Autodesk Inventor part; units mm, degrees
ref_plane "YZ Plane" through (0, 0, 0) normal (1, 0, 0) x (0, 1, 0)
ref_plane "XZ Plane" through (0, 0, 0) normal (0, 1, 0) x (-1, 0, 0)
ref_plane "XY Plane" through (0, 0, 0) normal (0, 0, 1) x (1, 0, 0)
sketch "Sketch1" plane through (0, 0, 0) normal (0, 0, 1) x (1, 0, 0)
  circle A0 centre (-11.375, 11.375) radius 2.1
  circle A1 centre (-11.375, -11.375) radius 2.1
  line L0 (-15, 4.1) -> (-12.9, 4.1)
  line L1 (-12.9, 4.1) -> (-12.9, 8.28)
  line L2 (-12.9, 8.28) -> (-9.85, 8.28)
  line L3 (-9.85, 8.28) -> (-5.8, 4.23)
  line L4 (-5.8, 4.23) -> (-5.8, -4.23)
  line L5 (-5.8, -4.23) -> (-9.85, -8.28)
  line L6 (-9.85, -8.28) -> (-12.9, -8.28)
  line L7 (-12.9, -8.28) -> (-12.9, -4.1)
  line L8 (-12.9, -4.1) -> (-15, -4.1)
  line L9 (-15, -4.1) -> (-15, -13)
  arc A2 (-15, -13) -> (-13, -15) centre (-13, -13) ccw
  line L10 (-13, -15) -> (-4.1, -15)
  line L11 (-4.1, -15) -> (-4.1, -12.9)
  line L12 (-4.1, -12.9) -> (-8.28, -12.9)
  line L13 (-8.28, -12.9) -> (-8.28, -9.85)
  line L14 (-8.28, -9.85) -> (-3.719, -5.289)
  line L15 (-3.719, -5.289) -> (3.719, -5.289)
  line L16 (3.719, -5.289) -> (8.28, -9.85)
  line L17 (8.28, -9.85) -> (8.28, -12.9)
  line L18 (8.28, -12.9) -> (4.1, -12.9)
  line L19 (4.1, -12.9) -> (4.1, -15)
  line L20 (4.1, -15) -> (13, -15)
  arc A3 (13, -15) -> (15, -13) centre (13, -13) ccw
  line L21 (15, -13) -> (15, -4.1)
  line L22 (15, -4.1) -> (12.9, -4.1)
  line L23 (12.9, -4.1) -> (12.9, -8.28)
  line L24 (12.9, -8.28) -> (9.85, -8.28)
  line L25 (9.85, -8.28) -> (5.8, -4.23)
  line L26 (5.8, -4.23) -> (5.8, 4.23)
  line L27 (5.8, 4.23) -> (9.85, 8.28)
  line L28 (9.85, 8.28) -> (12.9, 8.28)
  line L29 (12.9, 8.28) -> (12.9, 4.1)
  line L30 (12.9, 4.1) -> (15, 4.1)
  line L31 (15, 4.1) -> (15, 13)
  arc A4 (15, 13) -> (13, 15) centre (13, 13) ccw
  line L32 (13, 15) -> (4.1, 15)
  line L33 (4.1, 15) -> (4.1, 12.9)
  line L34 (4.1, 12.9) -> (8.28, 12.9)
  line L35 (8.28, 12.9) -> (8.28, 9.85)
  line L36 (8.28, 9.85) -> (3.719, 5.289)
  line L37 (3.719, 5.289) -> (-3.719, 5.289)
  line L38 (-3.719, 5.289) -> (-8.28, 9.85)
  line L39 (-8.28, 9.85) -> (-8.28, 12.9)
  line L40 (-8.28, 12.9) -> (-4.1, 12.9)
  line L41 (-4.1, 12.9) -> (-4.1, 15)
  line L42 (-4.1, 15) -> (-13, 15)
  arc A5 (-13, 15) -> (-15, 13) centre (-13, 13) ccw
  line L43 (-15, 13) -> (-15, 4.1)
  circle A6 centre (0, 0) radius 3.4
  circle A7 centre (11.375, 11.375) radius 2.1
  circle A8 centre (11.375, -11.375) radius 2.1
extrude "Extrusion1" add sketch "Sketch1" against normal blind 300
sketch "Sketch2" plane through (-13, 15, 0) normal (0, 1, 0) x (1, 0, 0)
  point P0 (13, 0)
properties part number "Metal Profile 30 cm" material "Aluminum 6061-AHC"
The model under review builds one solid part; all positions refer to its coordinate system, in mm. A direction names the side the tool comes from. Coordinates: 2 decimals unless noted, no trailing zeros. Write each loop counter-clockwise with the first axis right and the second up, starting at its lowest first coordinate (ties: lowest second). Pieces come first, ordered by that corner, then holes. Notation, with made-up numbers: (-13.75, 68.5) - (23.25, 68.5) arc R9 ccw to (23.25, 78.5) - close; hole circle Ø9 at (64.5, -18.5). An arc over 180 degrees is marked (long way). Answer in a Markdown table with one row per item. Add a question column.
Q1. Consider section A-A on x = 0. Give the boundary of the cut face in (y, z), then the cut area to 3 significant figures.
Q2. For faces 1 (the face through (0, -5.289, -148)), 2 (the face through (5.97, -7.54, -147.9)), 3 (the face through (9, 15, -148)), list the 3-axis set-ups (+Z, -Z, +X, -X, +Y, -Y) from which the entire face can be reached by the end or side of a thin tool; tool diameter is ignored.
Q3. Consider section C-C on z = -54.5. Give the number of separate pieces and of enclosed holes in the cut face, then the cut area to 3 significant figures.
Q4. To check wall thickness, follow line 1 along X through (y, z) = (11.5, -195.5); line 2 along X through (y, z) = (-0.25, -203); line 3 along Y through (x, z) = (0, -135). State the ranges of each line that lie inside material, in increasing order. Write a range as from..to.
Q5. Consider section B-B on y = 0. Give the boundary of the cut face in (x, z), then the cut area to 3 significant figures.
Q6. Clearance check with flat-ended pins moving along their axes: pin 1 (3.5 mm diameter, centred on x = 11.375, y = -11.375, fed in from -Z); pin 2 (2.5 mm diameter, centred on y = -14.5, z = -127, fed in from +X); pin 3 (1.7 mm diameter, centred on y = 14, z = -203, fed in from -X); pin 4 (4 mm diameter, centred on y = -0.5, z = -117.5, fed in from -X). State where each tip first meets the part, or that it passes through.
Q7. Draft analysis for pull direction X (two halves, no side actions). For faces 4 (the face through (-4, 0, 0)), 5 (the face through (15, 8, -148)), 6 (the face through (-15, 9, -148)), 7 (the face through (0, 5.289, -148)), state which applies: +X half, -X half, draft (parallel to the pull), parting line (faces both ways), or undercut.
Answers below:
| question | item | result |
|---|---|---|
| 1 | outline | (-5.29, -300) - (-3.4, -300) - (-3.4, 0) - (-5.29, 0) - close; (3.4, -300) - (5.29, -300) - (5.29, 0) - (3.4, 0) - close |
| 1 | area | 1,130 mm² |
| 2 | face 1 | +Z, -Z, -Y |
| 2 | face 2 | +Z, -Z |
| 2 | face 3 | +Z, -Z, +X, -X, +Y |
| 3 | separate pieces | 1 |
| 3 | enclosed holes | 5 |
| 3 | area | 323 mm² |
| 4 | line 1 | -15..-13.47, -9.28..-8.28, 8.28..9.28, 13.47..15 |
| 4 | line 2 | -5.8..-3.39, 3.39..5.8 |
| 4 | line 3 | -5.29..-3.4, 3.4..5.29 |
| 5 | outline | (-5.8, -300) - (-3.4, -300) - (-3.4, 0) - (-5.8, 0) - close; (3.4, -300) - (5.8, -300) - (5.8, 0) - (3.4, 0) - close |
| 5 | area | 1,440 mm² |
| 6 | pin 1 | through |
| 6 | pin 2 | x = 14.98 |
| 6 | pin 3 | x = -14.99 |
| 6 | pin 4 | x = -5.8 |
| 7 | face 4 | draft |
| 7 | face 5 | +X half |
| 7 | face 6 | -X half |
| 7 | face 7 | undercut |
